Input: part model. Units: mm. Frame: model coordinates. Round coordinates to 2 decimals unless told otherwise and drop trailing zeros. Loops run counter-clockwise (first coordinate to the right, second up) from the corner with the lowest first, then second, coordinate; pieces in that order, holes last. Notation, with made-up numbers: (44.25, 64.25) - (93.25, 64.25) arc R34 cw to (93.25, 100.25) - close; hole circle Ø10 at (29, 43.5). An arc over 180 degrees is marked (long way). One line per question, with ' | ' between items. Start each with the question number.
from build123d import *

# Parameters (mm, degrees)
SKETCH_1_W          = 25
SKETCH_1_H          = 10
SKETCH_1_R          = 1.6
EXTRUDE_1_DEPTH     = 10
CUT_EXTRUDE_1_REACH = 20.875
CUT_EXTRUDE_2_REACH = 20.875
SKETCH_4_R          = 2
CUT_EXTRUDE_3_DEPTH = 20.017855396
FILLET_1_R          = 4
FILLET_2_R          = 5


with BuildPart() as part:
    # ｽｹｯﾁ1 → ﾎﾞｽ - 押し出し1 (new body)
    with BuildSketch(Plane.XY):
        Rectangle(SKETCH_1_W, SKETCH_1_H)
        with Locations((-7.5, 0)):
            Circle(SKETCH_1_R, mode=Mode.SUBTRACT)
        with Locations((-2.5, 0)):
            Circle(SKETCH_1_R, mode=Mode.SUBTRACT)
    extrude(amount=EXTRUDE_1_DEPTH)

    # ｽｹｯﾁ2 → ｶｯﾄ - 押し出し1 (cut, up to next)
    with BuildSketch(Plane.XZ.offset(5), mode=Mode.PRIVATE) as cut_extrude_1_sk1:
        Polygon((2.5, 10), (10.5, 10), (2.5, 2), (-12.5, 2), (-12.5, 10), align=None)
    cut_extrude_1_tool1 = extrude(cut_extrude_1_sk1.sketch, amount=-CUT_EXTRUDE_1_REACH, mode=Mode.PRIVATE) & part.part
    # ｽｹｯﾁ2 → ｶｯﾄ - 押し出し1 (cut, up to next)
    with BuildSketch(Plane.XZ.offset(5), mode=Mode.PRIVATE) as cut_extrude_1_sk2:
        Polygon((3.328427125, 0), (12.5, 9.171572875), (12.5, 0), align=None)
    cut_extrude_1_tool2 = extrude(cut_extrude_1_sk2.sketch, amount=-CUT_EXTRUDE_1_REACH, mode=Mode.PRIVATE) & part.part
    add(cut_extrude_1_tool1.solids().sort_by_distance((-2.859649, -5, 6.280702))[0], mode=Mode.SUBTRACT)
    add(cut_extrude_1_tool2.solids().sort_by_distance((9.442809, -5, 3.057191))[0], mode=Mode.SUBTRACT)

    # ｽｹｯﾁ3 → ｶｯﾄ - 押し出し2 (cut, up to next)
    with BuildSketch(Plane.XZ.offset(5), mode=Mode.PRIVATE) as cut_extrude_2_sk1:
        Polygon((10.5, 10), (11.914213562, 8.585786438), (12.5, 9.171572875), (12.5, 10), align=None)
    cut_extrude_2_tool1 = extrude(cut_extrude_2_sk1.sketch, amount=-CUT_EXTRUDE_2_REACH, mode=Mode.PRIVATE) & part.part
    add(cut_extrude_2_tool1.solids().sort_by_distance((11.735702, -5, 9.488155))[0], mode=Mode.SUBTRACT)

    # ｽｹｯﾁ4 → ｶｯﾄ - 押し出し3 (cut, through all)
    with BuildSketch(Plane(origin=(1.664213562, 0, -1.664213562), x_dir=(-0.7071067811865509, 0, -0.7071067811865441), z_dir=(0.7071067811865441, 0, -0.7071067811865509))):
        with Locations((-11.203553391, 0)):
            Circle(SKETCH_4_R)
    extrude(amount=-CUT_EXTRUDE_3_DEPTH, mode=Mode.SUBTRACT)

    # ﾌｨﾚｯﾄ1
    fillet_1_edges = [part.edges().sort_by_distance(p)[0] for p in [
        (3.328427125, 0, 0),
        (2.5, 0, 2),
    ]]
    fillet(fillet_1_edges, radius=FILLET_1_R)

    # ﾌｨﾚｯﾄ2
    fillet_2_edges = [part.edges().sort_by_distance(p)[0] for p in [
        (11.207106781, 5, 9.292893219),
        (11.207106781, -5, 9.292893219),
        (-12.5, -5, 1),
        (-12.5, 5, 1),
    ]]
    fillet(fillet_2_edges, radius=FILLET_2_R - 0.0001)  # a hair under: the kernel refuses the full size


solid = part.part
(1) Line query: line 1 along X through (y, z) = (0, 1.2); line 2 along Y through (x, z) = (-2.5, 1.15); line 3 along Z through (x, y) = (-9, 2.5). Output: solid intervals per line, ascending. Write a range as from..to.
(2) Section B-B, the plane y = -0.5. Output: boundary loops of the cut face in (x, z), plus the area to 3 significant figures.
(3) Section C-C, the plane y = 3. Output: boundary loops of the cut face in (x, z), plus the area to 3 significant figures.
(4) Pull-direction query (X, two-part tool) for faces 1 (the face through (-11.07, -3.5, 1.01)), 2 (the face through (-0.974, 0.481, 0.986)), 3 (the face through (-5.7, -0.1, 2)); classes: released by +X, released by -X, zero draft, split by the parting line, or undercut.
(5) Pin query (flat end, axial travel): P1, Ø1, axis at x = 9, y = -1, coming from the -Z side; P2, Ø5, axis at x = -4.5, y = 1.5, coming from the +Z side; P3, Ø5, axis at y = -3, z = 6, coming from the +X side. Return the tip coordinate at first contact, or that it passes through.
(6) Section D-D, the plane x = 5.75. Output: boundary loops of the cut face in (y, z), plus the area to 3 significant figures.
(7) Section A-A, the plane x = -2.5. Output: boundary loops of the cut face in (y, z).
Derived:
1) line 1: x = -12.5..-9.1, -5.9..-4.1, -0.9..4.53 | line 2: y = -5..-1.6, 1.6..5 | line 3: z = 0..2
2) outline: (-12.47, 0) - (-9.02, 0) - (-9.02, 2) - (-12.47, 2) - close; (-5.98, 0) - (-4.02, 0) - (-4.02, 2) - (-5.98, 2) - close; (-0.98, 0) - (1.67, 0) arc R4 ccw to (4.5, 1.17) - (8.22, 4.89) - (6.8, 6.3) - (3.67, 3.17) arc R4 cw to (0.84, 2) - (-0.98, 2) - close; (9.54, 9.04) - (10.96, 7.63) - (11.9, 8.57) - (10.48, 9.98) - close | area: 34.3 mm²
3) outline: (-11.5, 0) - (1.67, 0) arc R4 ccw to (4.5, 1.17) - (11.21, 7.88) - (9.79, 9.29) - (3.67, 3.17) arc R4 cw to (0.84, 2) - (-11.5, 2) - close | area: 50.3 mm²
4) face 1: released by -X | face 2: undercut | face 3: zero draft
5) P1: stops at z = 8.56 | P2: stops at z = 2 | P3: stops at x = 11.62
6) outline: (-5, 2.42) - (5, 2.42) - (5, 5.25) - (-5, 5.25) - close | area: 28.3 mm²
7) outline: (-5, 0) - (-1.6, 0) - (-1.6, 2) - (-5, 2) - close; (1.6, 0) - (5, 0) - (5, 2) - (1.6, 2) - close
